For this review, take the finished solid that the model builds, in its own axes (mm). Face numbers are marked on the shaded views. A direction names the side the tool comes from. Coordinates: 2 decimals unless noted, no trailing zeros. Write each loop counter-clockwise with the first axis right and the second up, starting at its lowest first coordinate (ties: lowest second). Pieces come first, ordered by that corner, then holes.
1) We need section D-D on y = 6. Write out the cut boundary in (x, z), then the cut area to 3 significant figures.
2) Mouldability with a two-part tool opening along X and no side actions: class the marked faces 1, 2 and 3 as pulls with the +X half, pulls with the -X half, needs draft (parallel to the pull), parting line crosses it, or undercut.
3) To check wall thickness, follow line 1 along X through (y, z) = (72, -11); line 2 along Z through (x, y) = (9, 13); line 3 along Y through (x, z) = (54, 14.5). State the ranges of each line that lie inside material, in increasing order.
4) We need section A-A on y = 72.5. Write out the cut boundary in (x, z).
5) We need section C-C on z = -27.5. Write out the cut boundary in (x, y), then the cut area to 3 significant figures.
6) For the marked faces 4, 5, 6 and 7, list the 3-axis set-ups (+Z, -Z, +X, -X, +Y, -Y) from which the entire face can be reached by the end or side of a thin tool; tool diameter is ignored.
7) Insertion check: P1, Ø4.5, axis at y = 66.5, z = -32, coming from the +X side; P2, Ø5, axis at x = 58, z = -6, coming from the +Y side; P3, Ø9.5, axis at x = 90.5, z = 20, coming from the -Y side. Each pin has a flat end and moves straight along its axis. Give the tip position at first contact, or say it passes through.
8) We need section B-B on x = 111. Write out the cut boundary in (y, z).
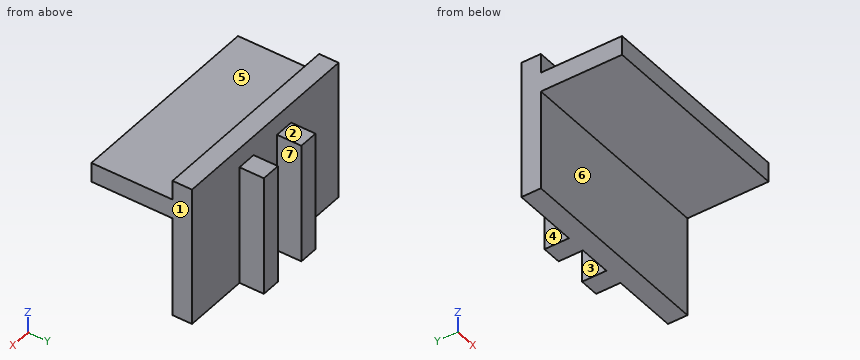
from build123d import *

# Parameters (mm, degrees)
SKETCH1_W           = 125
SKETCH1_H           = 62
BOSS_EXTRUDE2_DEPTH = 12
SKETCH3_W           = 125
SKETCH3_H           = 62
BOSS_EXTRUDE3_DEPTH = 12
SKETCH4_W           = 12
SKETCH4_H           = 74
BOSS_EXTRUDE4_DEPTH = 15
SKETCH5_W           = 125
SKETCH5_H           = 12
BOSS_EXTRUDE5_DEPTH = 12


with BuildPart() as part:
    # Sketch1 → Boss-Extrude2 (new body)
    with BuildSketch(Plane.XY):
        with Locations((62.5, 31)):
            Rectangle(SKETCH1_W, SKETCH1_H)
    extrude(amount=BOSS_EXTRUDE2_DEPTH)

    # Sketch3 → Boss-Extrude3 (add)
    with BuildSketch(Plane(origin=(0, 62, 0), x_dir=(1, 0, 0), z_dir=(0, 1, 0))):
        with Locations((62.5, 31)):
            Rectangle(SKETCH3_W, SKETCH3_H)
    extrude(amount=-BOSS_EXTRUDE3_DEPTH)

    # Sketch4 → Boss-Extrude4 (add)
    with BuildSketch(Plane(origin=(0, 62, 0), x_dir=(1, 0, 0), z_dir=(0, 1, 0))):
        with Locations((46.5, 25)):
            Rectangle(SKETCH4_W, SKETCH4_H)
        with Locations((78.5, 25)):
            Rectangle(SKETCH4_W, SKETCH4_H)
    extrude(amount=BOSS_EXTRUDE4_DEPTH)

    # Sketch5 → Boss-Extrude5 (add)
    with BuildSketch(Plane.XY.offset(12)):
        with Locations((62.5, 56)):
            Rectangle(SKETCH5_W, SKETCH5_H)
    extrude(amount=BOSS_EXTRUDE5_DEPTH)


solid = part.part
Result:
1. outline: (0, 0) - (125, 0) - (125, 12) - (0, 12) - close
1. area: 1,500 mm2
2. face 1: pulls with the +X half
2. face 2: needs draft
2. face 3: undercut
3. line 1: x = 40.5 to 52.5, 72.5 to 84.5
3. line 2: z = 0 to 12
3. line 3: y = 50 to 62
4. outline: (40.5, -62) - (52.5, -62) - (52.5, 12) - (40.5, 12) - close; (72.5, -62) - (84.5, -62) - (84.5, 12) - (72.5, 12) - close
5. outline: (0, 50) - (125, 50) - (125, 62) - (84.5, 62) - (84.5, 77) - (72.5, 77) - (72.5, 62) - (52.5, 62) - (52.5, 77) - (40.5, 77) - (40.5, 62) - (0, 62) - close
5. area: 1,860 mm2
6. face 4: +Z, -Z, -X, +Y
6. face 5: +Z, +X, -X, -Y
6. face 6: -Z, +X, -X, -Y
6. face 7: +Z, -Z, +Y
7. P1: stops at x = 84.5
7. P2: stops at y = 62
7. P3: stops at y = 50
8. outline: (0, 0) - (50, 0) - (50, -62) - (62, -62) - (62, 24) - (50, 24) - (50, 12) - (0, 12) - close
